For this review, take the finished solid that the model builds, in its own axes (mm). A direction names the side the tool comes from. Give positions to 0.01 mm unless a question says otherwise; leave off trailing zeros. Order: outer loops, then holes, each group sorted by start corner. A loop starts at its lowest first (then second) coordinate and runs counter-clockwise, first axis right, second up. Notation, with made-up numbers: (40.5, 18) - (64.5, 18) arc R18 ccw to (64.5, 35) - close; hole circle Ø8 at (78.25, 73.25). An arc over 180 degrees is marked (long way). One line per item, written item: value.
```python
from build123d import *

# Parameters (mm, degrees)
F0_R     = 16.5
F1_DEPTH = 9
F4_R     = 19
F5_DEPTH = 2.5
F2_R     = 15.5
F6_DEPTH = 6.6


# Not quite as in the source:
# - a fillet or chamfer that OpenCascade refuses, or shapes differently, is made with other operations: its cross-section is extruded or revolved along the edge and cut away or added


with BuildPart() as f1:
    # F0 (on Top) → F1 (new body)
    with BuildSketch(Plane.XY):
        Circle(F0_R)
    extrude(amount=F1_DEPTH)

    # F4 (on offset) → F5 (join)
    with BuildSketch(Plane.XY.offset(5.5)):
        Circle(F4_R)
    extrude(amount=-F5_DEPTH)

    # F2 (on face) → F6 (cut)
    with BuildSketch(Plane.XY.offset(9)):
        Circle(F2_R)
    extrude(amount=-F6_DEPTH, mode=Mode.SUBTRACT)

    # F7: fillet of radius 3 on 1 edges, made by hand

    # F7_s1 → F7_t2 (revolve)
    with BuildSketch(Plane.XZ):
        with BuildLine():
            ThreePointArc((16.5, 0.0419601084), (17.2087121525, 1.9784517816), (19, 3))
            Line((19, 3), (16.5, 3))
            Line((16.5, 3), (16.5, 0.0419601084))
        make_face()
    revolve(axis=Axis((0, 0, 3), (0, 0, -1)))


solid = f1.part
```
(1) For P1, Ø9.5, axis at x = -0.5, y = 6.5, coming from the +Z side; P2, Ø4, axis at x = 13.5, y = 2, coming from the +Z side; P3, Ø3, axis at y = -2, z = 5.5, coming from the +X side; P4, Ø1.5, axis at y = -13, z = 4.5, coming from the +X side, all flat-tipped, find the tip position at first contact; note any pin that passes through.
Answers below:
P1: stops at z = 2.4
P2: stops at z = 9
P3: stops at x = 18.99
P4: stops at x = 14.52
(2) Take a section at A-A (x = 0). Write out the cut boundary in (y, z), then the cut area to 3 significant figures.
Answers below:
outline: (-19, 3) arc R3 cw to (-16.5, 0.04) - (-16.5, 0) - (16.5, 0) - (16.5, 0.04) arc R3 cw to (19, 3) - (19, 5.5) - (16.5, 5.5) - (16.5, 9) - (15.5, 9) - (15.5, 2.4) - (-15.5, 2.4) - (-15.5, 9) - (-16.5, 9) - (-16.5, 5.5) - (-19, 5.5) - close
area: 109 mm^2
(3) Machinability: for faces 5 (the face through (-6, 16, 5.5)), 6 (the face through (8.767, -16.856, 4.268)), which of the approach directions +Z, -Z, +X, -X, +Y, -Y give a long, thin tool a straight path to every point of the face, cutting with its end or side? Answer none if there is none.
Answers below:
face 5: +Z
face 6: +Z, -Z
(4) Wall thickness on line 1 (Y direction, x = 0, z = 5); line 2 (Y direction, x = 0, z = 7.75); line 3 (Z direction, x = -2, y = -0.5): over which ranges is each line inside the solid? List them lowest first. Write a range as from..to.
Answers below:
line 1: y = -19..-15.5, 15.5..19
line 2: y = -16.5..-15.5, 15.5..16.5
line 3: z = 0..2.4
(5) Take a section at C-C (z = 3.5). Write out the cut boundary in (x, y), then the cut area to 3 significant figures.
Answers below:
outline: circle Ø38 at (0, 0); hole circle Ø31 at (0, 0)
area: 379 mm^2
(6) Draft analysis for pull direction X (two halves, no side actions). For faces 1 (the face through (15.24, -6.32, 7.23)), 2 (the face through (-2.018, 15.368, 5.746)), 3 (the face through (0, 0, 0)), 4 (the face through (0, 0, 2.4)), state which applies: pulls with the +X half, pulls with the -X half, needs draft (parallel to the pull), parting line crosses it, or undercut.
Answers below:
face 1: parting line crosses it
face 2: undercut
face 3: needs draft
face 4: undercut
